Part print with two shaded views. Sizes in mm from the minimum x, y, z corner. Round coordinates to 2 decimals unless told otherwise and drop trailing zeros. Order: outer loops, then holes, each group sorted by start corner. A loop starts at its lowest first (then second) coordinate and runs counter-clockwise, first axis right, second up. Notation, with made-up numbers: M 32,14 L 72,14 A13 cw 72,39 Z; hole C 45,58 d11. An arc over 180 degrees is marked long. Put each result on its own line as item: value.
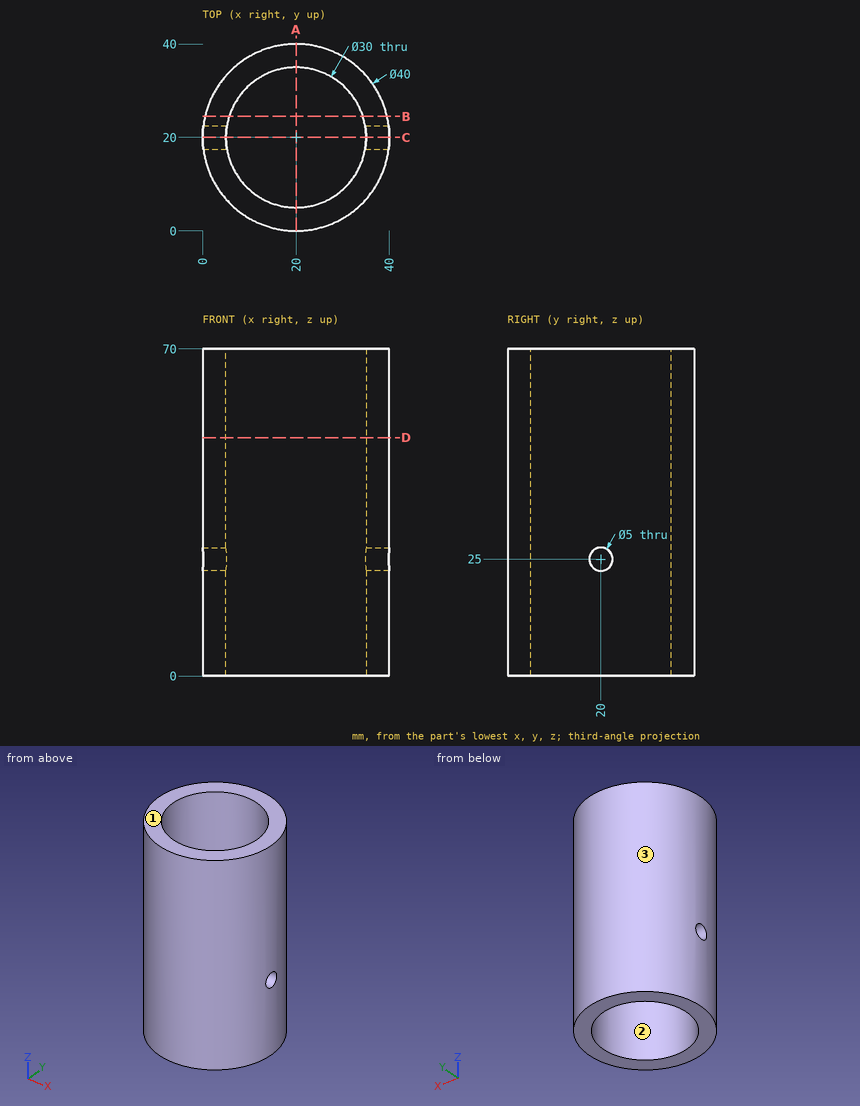
Item 1: Mould opens along Y. For the marked faces 1, 2 and 3 say: pulls with the +Y half, pulls with the -Y half, needs draft (parallel to the pull), parting line crosses it, or undercut.
Answers below:
face 1: needs draft
face 2: undercut
face 3: parting line crosses it
Item 2: Probe line 1 along Y through (x, z) = (20, 38); line 2 along X through (y, z) = (20.5, 40); line 3 along Y through (x, z) = (18, 51.5). List the from-to ranges inside material, lowest first. Write a range as [from, to].
Answers below:
line 1: [0, 5], [35, 40]
line 2: [0.01, 5.01], [34.99, 39.99]
line 3: [0.1, 5.13], [34.87, 39.9]
Item 3: Pin check, flat tips, straight feed: P1, Ø12, axis at y = 30, z = 23.5, coming from the +X side; P2, Ø1, axis at x = 14, z = 36, coming from the +Y side; P3, Ø4, axis at x = 28.5, z = 55, coming from the +Y side; P4, Ø3, axis at y = 20, z = 25, coming from the -X side. Stop position of each tip, or through.
Answers below:
P1: x = 39.6
P2: y = 39.23
P3: y = 38.91
P4: through
Item 4: Band-saw the part on A-A on x = 20. Give the cut face in (y, z), and give its area (3 significant figures).
Answers below:
outline: M 0,0 L 5,0 L 5,70 L 0,70 Z; M 35,0 L 40,0 L 40,70 L 35,70 Z
area: 700 mm²
Item 5: Band-saw the part on D-D on z = 51. Give the cut face in (x, y), and give its area (3 significant figures).
Answers below:
outline: C 20,20 d40; hole C 20,20 d30
area: 550 mm²
Item 6: Band-saw the part on C-C on y = 20. Give the cut face in (x, z), and give its area (3 significant figures).
Answers below:
outline: M 0,0 L 5,0 L 5,22.5 L 0,22.5 Z; M 0,27.5 L 5,27.5 L 5,70 L 0,70 Z; M 35,0 L 40,0 L 40,22.5 L 35,22.5 Z; M 35,27.5 L 40,27.5 L 40,70 L 35,70 Z
area: 650 mm²
Item 7: Band-saw the part on B-B on y = 24.5. Give the cut face in (x, z).
Answers below:
outline: M 0.51,0 L 5.69,0 L 5.69,70 L 0.51,70 Z; M 34.31,0 L 39.49,0 L 39.49,70 L 34.31,70 Z
